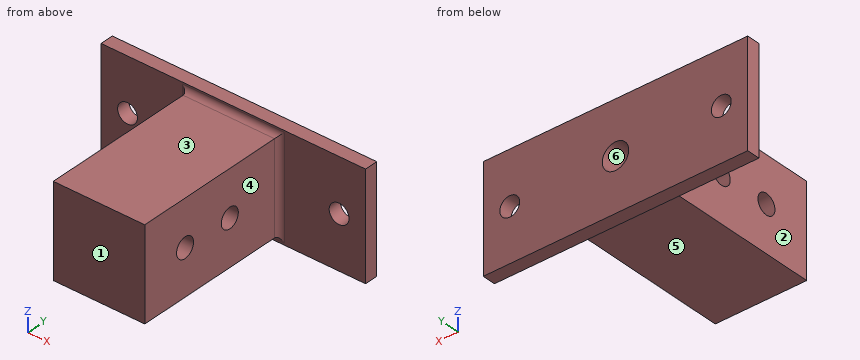
```python
from build123d import *

# Parameters (mm, degrees)
SKETCH1_W           = 21.971
SKETCH1_H           = 21.971
BOSS_EXTRUDE1_DEPTH = 38.1
SKETCH2_W           = 63.5
SKETCH2_H           = 25.4
BOSS_EXTRUDE2_DEPTH = 3.175
SKETCH3_R           = 2.38125
CUT_EXTRUDE1_DEPTH  = 3.175
FILLET1_R           = 1.27
SKETCH4_R           = 3.175
CUT_EXTRUDE2_DEPTH  = 15.24
SKETCH5_R           = 2.413
CUT_EXTRUDE3_DEPTH  = 25.4


with BuildPart() as part:
    # Sketch1 → Boss-Extrude1 (new body)
    with BuildSketch(Plane(origin=(0, 0, 0), x_dir=(1, 0, 0), z_dir=(0, 1, 0))):
        Rectangle(SKETCH1_W, SKETCH1_H)
    extrude(amount=BOSS_EXTRUDE1_DEPTH)

    # Sketch2 → Boss-Extrude2 (add)
    with BuildSketch(Plane(origin=(0, 38.1, 0), x_dir=(1, 0, 0), z_dir=(0, 1, 0))):
        Rectangle(SKETCH2_W, SKETCH2_H)
    extrude(amount=BOSS_EXTRUDE2_DEPTH)

    # Sketch3 → Cut-Extrude1 (cut)
    with BuildSketch(Plane(origin=(0, 41.275, 0), x_dir=(1, 0, 0), z_dir=(0, 1, 0))):
        with Locations(Location((25.4, 0, 0), (0, 0, 270))):
            Circle(SKETCH3_R)
        with Locations(Location((-25.4, 0, 0), (0, 0, 270))):
            Circle(SKETCH3_R)
    extrude(amount=-CUT_EXTRUDE1_DEPTH, mode=Mode.SUBTRACT)

    # Fillet1
    fillet1_edges = [part.edges().sort_by_distance(p)[0] for p in [
        (-10.9855, 38.1, 0),
        (0, 38.1, 10.9855),
        (10.9855, 38.1, 0),
        (0, 38.1, -10.9855),
    ]]
    fillet(fillet1_edges, radius=FILLET1_R)

    # Sketch4 → Cut-Extrude2 (cut)
    with BuildSketch(Plane(origin=(0, 41.275, 0), x_dir=(1, 0, 0), z_dir=(0, 1, 0))):
        with Locations(Location((0, 0, 0), (0, 0, 270))):
            Circle(SKETCH4_R)
    extrude(amount=-CUT_EXTRUDE2_DEPTH, mode=Mode.SUBTRACT)

    # Sketch5 → Cut-Extrude3 (cut)
    with BuildSketch(Plane(origin=(10.9855, 0, 0), x_dir=(0, 0, -1), z_dir=(1, 0, 0))):
        with Locations((0, 24.13)):
            Circle(SKETCH5_R)
        with Locations((0, 11.43)):
            Circle(SKETCH5_R)
    extrude(amount=-CUT_EXTRUDE3_DEPTH, mode=Mode.SUBTRACT)


solid = part.part
```
Check sheet for the modelled part. Datum: model origin and axes. Units: mm. Face numbers are marked on the shaded views. A direction names the side the tool comes from. Coordinates: 2 decimals unless noted, no trailing zeros. Write each loop counter-clockwise with the first axis right and the second up, starting at its lowest first coordinate (ties: lowest second). Pieces come first, ordered by that corner, then holes. Notation, with made-up numbers: (50.25, -18.75) -> (63.25, -18.75) arc R17 ccw to (63.25, -11.75) -> close; hole circle Ø4 at (65.5, -29.5). An arc over 180 degrees is marked (long way). Use a Markdown table: item, result.
1. Release check for a two-part mould opening along Z. For the marked faces 4, 5 and 6 record: pulls with the +Z half, pulls with the -Z half, needs draft (parallel to the pull), parting line crosses it, or undercut.
Reported:
| item | result |
|---|---|
| face 4 | needs draft |
| face 5 | pulls with the -Z half |
| face 6 | undercut |
2. Scan lines: line 1 along Y through (x, z) = (-5.5, 0) (3 decimals); line 2 along X through (y, z) = (39.85, 0) (3 decimals); line 3 along X through (y, z) = (35.5, 0) (1 decimal). Record each from-to range of solid material in increasing order.
Reported:
| item | result |
|---|---|
| line 1 | y = 0 to 9.017, 13.843 to 21.717, 26.543 to 41.275 |
| line 2 | x = -31.75 to -27.781, -23.019 to -3.175, 3.175 to 23.019, 27.781 to 31.75 |
| line 3 | x = -11 to -3.2, 3.2 to 11 |
3. Sectioned sample at D-D (x = 0). Enter the section's corners in (y, z) (1 decimal), plus the area to 3 significant figures.
Reported:
| item | result |
|---|---|
| outline | (0, -11) -> (36.8, -11) arc R1.3 cw to (38.1, -12.3) -> (38.1, -12.7) -> (41.3, -12.7) -> (41.3, -3.2) -> (26, -3.2) -> (26, -1.5) arc R2.4 cw (long way) to (26, 1.5) -> (26, 3.2) -> (41.3, 3.2) -> (41.3, 12.7) -> (38.1, 12.7) -> (38.1, 12.3) arc R1.3 cw to (36.8, 11) -> (0, 11) -> close; hole circle Ø4.8 at (11.4, 0) |
| area | 786 mm2 |
4. Sectioned sample at B-B (x = 25.4). Enter the section's corners in (y, z) (3 decimals).
Reported:
| item | result |
|---|---|
| outline | (38.1, -12.7) -> (41.275, -12.7) -> (41.275, -2.381) -> (38.1, -2.381) -> close; (38.1, 2.381) -> (41.275, 2.381) -> (41.275, 12.7) -> (38.1, 12.7) -> close |
5. Go/stop test with flat-tipped pins: pin 1 Ø5.5 at (y, z) = (11.43, 0) entering from +X; pin 2 Ø8 at (y, z) = (37, -10) entering from -X; pin 3 Ø6.5 at (y, z) = (14.5, 0.5) entering from -X; pin 4 Ø6.5 at (x, y) = (-2.5, 23.5) entering from -Z. Record where each tip stops, or that it passes through.
Reported:
| item | result |
|---|---|
| pin 1 | stops at x = 10.99 |
| pin 2 | stops at x = -31.75 |
| pin 3 | stops at x = -10.99 |
| pin 4 | stops at z = -10.99 |
6. Sectioned sample at C-C (y = 24.13). Enter the section's corners in (x, z).
Reported:
| item | result |
|---|---|
| outline | (-10.99, -10.99) -> (10.99, -10.99) -> (10.99, -2.41) -> (-10.99, -2.41) -> close; (-10.99, 2.41) -> (10.99, 2.41) -> (10.99, 10.99) -> (-10.99, 10.99) -> close |
7. Tool access check on the marked faces 1, 2 and 3. Record the directions out of +Z, -Z, +X, -X, +Y, -Y that give a thin tool (end or side, any length) a straight path to the whole face; none if there is none.
Reported:
| item | result |
|---|---|
| face 1 | +Z, -Z, +X, -X, -Y |
| face 2 | +Z, -Z, -X, -Y |
| face 3 | +Z, +X, -X, -Y |
8. Sectioned sample at A-A (z = 0). Give the number of separate pieces and of enclosed holes in the cut face, plus the area to 3 significant figures.
Reported:
| item | result |
|---|---|
| separate pieces | 6 |
| enclosed holes | 0 |
| area | 704 mm2 |
